from build123d import *

# Parameters (mm, degrees)
SKETCH1_R           = 2.5
BOSS_EXTRUDE1_DEPTH = 30
DRAFT2_ANGLE        = 1
DRAFT4_ANGLE        = -1


with BuildPart() as part:
    # Sketch1 → Boss-Extrude1 (new body)
    with BuildSketch(Plane.XY):
        Circle(SKETCH1_R)
    extrude(amount=BOSS_EXTRUDE1_DEPTH)

    # Draft2
    draft2_faces = [part.faces().sort_by_distance(p)[0] for p in [
        (-2.5, 0, 15),
    ]]
    draft(draft2_faces, Plane(origin=(0, 0, 0), x_dir=(-1, 0, 0), z_dir=(0, 0, -1)), DRAFT2_ANGLE)

    # Draft4
    draft4_faces = [part.faces().sort_by_distance(p)[0] for p in [
        (-2.761825974, 0, 15),
    ]]
    draft(draft4_faces, Plane(origin=(0, 0, 0), x_dir=(-1, 0, 0), z_dir=(0, 0, -1)), DRAFT4_ANGLE)


solid = part.part
Build history of the part. All positions in model axes, mm. A direction names the side the tool comes from. Round coordinates to 2 decimals unless told otherwise and drop trailing zeros. Loops run counter-clockwise (first coordinate to the right, second up) from the corner with the lowest first, then second, coordinate; pieces in that order, holes last. Notation, with made-up numbers: (-36, 87.5) -> (15, 87.5) arc R21 ccw to (15, 110.5) -> close; hole circle Ø9 at (59.5, 6.25). An arc over 180 degrees is marked (long way). Use CSV: the item, a comma, the result in double quotes. Start each with the question number.
Q1. Saw through at B-B on z = 15. Give the cut face in (x, y).
Q2. Saw through at A-A on z = 19. Give the cut face in (x, y).
Q3. Drill centre lines: L1, parallel to X at y = -1.05, z = 24; L2, parallel to X at y = 1.75, z = 3.5; L3, parallel to Y at x = 0.55, z = 27. Where is each one in solid material? Low to high.
Q4. Which spindle directions (+Z, -Z, +X, -X, +Y, -Y) get a long thin tool onto all of the face, cutting with end or side? Do faces 1 (the face through (-1.78, -1.36, 14.79)), 2 (the face through (0, 0, 0)). Say none if no direction does.
Q5. Flat gauge pins, fed straight in: pin 1 Ø3 at (x, y) = (1, -1.5) entering from -Z; pin 2 Ø1.5 at (y, z) = (-0.5, 17.5) entering from -X; pin 3 Ø2 at (x, z) = (-1.5, 11) entering from +Y; pin 4 Ø3 at (x, z) = (0.5, 10.5) entering from -Y. Where does each tip first touch, or does it go through?
Solutions:
1,outline,"circle Ø4.48 at (0, 0)"
2,outline,"circle Ø4.34 at (0, 0)"
3,L1,"x = -1.8 to 1.8"
3,L2,"x = -1.7 to 1.7"
3,L3,"y = -1.95 to 1.95"
4,face 1,"+Z"
4,face 2,"-Z, +X, -X, +Y, -Y"
5,pin 1,"stops at z = 0"
5,pin 2,"stops at x = -2.2"
5,pin 3,"stops at y = 2.25"
5,pin 4,"stops at y = -2.34"
